from build123d import *

# Parameters (mm, degrees)
F0_R     = 35
F0_R_2   = 2.5
F1_DEPTH = 5
F2_R     = 10
F3_DEPTH = 20
F4_R     = 7.5
F5_DEPTH = 60
F6_R     = 2.5
F7_SIZE  = 1


with BuildPart() as f1:
    # F0 (on Top) → F1 (new body)
    with BuildSketch(Plane.XY):
        Circle(F0_R)
        with Locations((-20.7846096908, -12.3947781175)):
            Circle(F0_R_2, mode=Mode.SUBTRACT)
        with Locations((0, -24.3947781175)):
            Circle(F0_R_2, mode=Mode.SUBTRACT)
        with Locations((20.7846096908, -12.3947781175)):
            Circle(F0_R_2, mode=Mode.SUBTRACT)
        with Locations((-20.7846096908, 11.6052218825)):
            Circle(F0_R_2, mode=Mode.SUBTRACT)
        with Locations((20.7846096908, 11.6052218825)):
            Circle(F0_R_2, mode=Mode.SUBTRACT)
        with Locations((0, 23.6052218825)):
            Circle(F0_R_2, mode=Mode.SUBTRACT)
    extrude(amount=F1_DEPTH)

    # F2 (on Top) → F3 (join)
    with BuildSketch(Plane.XY):
        Circle(F2_R)
    extrude(amount=F3_DEPTH)

    # F4 (on Top) → F5 (join)
    with BuildSketch(Plane.XY):
        Circle(F4_R)
    extrude(amount=F5_DEPTH)

    # F6
    f6_edges = [f1.edges().sort_by_distance(p)[0] for p in [
        (-10, 0, 5),
    ]]
    fillet(f6_edges, radius=F6_R)

    # F7
    f7_edges = [f1.edges().sort_by_distance(p)[0] for p in [
        (-10, 0, 20),
    ]]
    chamfer(f7_edges, length=F7_SIZE)


solid = f1.part
Could you check a few things on this model? Use its own coordinates, in mm. A direction names the side the tool comes from. Round coordinates to 2 decimals unless told otherwise and drop trailing zeros. Write each loop counter-clockwise with the first axis right and the second up, starting at its lowest first coordinate (ties: lowest second). Pieces come first, ordered by that corner, then holes. Notation, with made-up numbers: (69.5, 36) - (103.5, 36) arc R17 cw to (103.5, 61) - close; hole circle Ø5 at (83.5, 75.25). An arc over 180 degrees is marked (long way). Put each result on its own line as item: value. Start each with the question number.
(1) I want a section at D-D, the plane x = 28. Please give me the cut outline in (y, z), plus the area to 3 significant figures.
(2) I need wall thicknesses on probe 1 along Y at (x, z) = (0, 1.55); probe 2 along Z at (x, y) = (-3, 19); probe 3 along Y at (x, z) = (2, 26). Which ranges of each line are inside material? Lowest first, please.
(3) For faces 5 (the cylindrical face through (-18.475, 10.648, 2.465)), 6 (the flat face through (0, -15, 5)), which set-ups out of +Z, -Z, +X, -X, +Y, -Y let a thin tool reach every point of the face, with its end or its side?
(4) I want a section at C-C, the plane z = 35. Please give me the cut outline in (x, y).
(5) I want a section at A-A, the plane x = 0. Please give me the cut outline in (y, z).
(6) Will these pins go through, and if not, where does the flat tip stop? pin 1 (8 mm diameter, centred on x = 3, y = 20.5, fed in from +Z); pin 2 (6 mm diameter, centred on x = -25, y = -17.5, fed in from -Z); pin 3 (2 mm diameter, centred on x = 7, z = 14, fed in from -Y); pin 4 (4 mm diameter, centred on x = -6, z = 11.5, fed in from -Y).
(7) Thinking about a two-plate mould opening in Y: for faces 1 (the cylindrical face through (-7.493, 0.33, 39.72)), 2 (the cylindrical face through (18.287, -12.285, 2.465)), 3 (the flat face through (-2, 7.4, 20)), 4 (the cylindrical face through (1.154, 21.387, 2.465)), which applies, released by +Y, released by -Y, zero draft, split by the parting line, or undercut?
(8) I want a section at B-B, the plane y = 0. Please give me the cut outline in (x, z).
Here are the results:
1. outline: (-21, 0) - (21, 0) - (21, 5) - (-21, 5) - close
1. area: 210 mm^2
2. probe 1: y = -35 to -26.89, -21.89 to 21.11, 26.11 to 35
2. probe 2: z = 0 to 5
2. probe 3: y = -7.23 to 7.23
3. face 5: +Z, -Z
3. face 6: +Z
4. outline: circle Ø15 at (0, 0)
5. outline: (-35, 0) - (-26.89, 0) - (-26.89, 5) - (-35, 5) - close; (-21.89, 0) - (21.11, 0) - (21.11, 5) - (12.5, 5) arc R2.5 cw to (10, 7.5) - (10, 19) - (9, 20) - (7.5, 20) - (7.5, 60) - (-7.5, 60) - (-7.5, 20) - (-9, 20) - (-10, 19) - (-10, 7.5) arc R2.5 cw to (-12.5, 5) - (-21.89, 5) - close; (26.11, 0) - (35, 0) - (35, 5) - (26.11, 5) - close
6. pin 1: stops at z = 5
6. pin 2: stops at z = 0
6. pin 3: stops at y = -8
6. pin 4: stops at y = -9.17
7. face 1: split by the parting line
7. face 2: undercut
7. face 3: zero draft
7. face 4: undercut
8. outline: (-35, 0) - (35, 0) - (35, 5) - (12.5, 5) arc R2.5 cw to (10, 7.5) - (10, 19) - (9, 20) - (7.5, 20) - (7.5, 60) - (-7.5, 60) - (-7.5, 20) - (-9, 20) - (-10, 19) - (-10, 7.5) arc R2.5 cw to (-12.5, 5) - (-35, 5) - close
